Read the model definition and answer for the solid it produces. Units are mm, in the model's axes. A direction names the side the tool comes from. Give positions to 0.01 mm unless a question says otherwise; leave off trailing zeros. Order: outer loops, then holes, each group sorted by start corner. A loop starts at its lowest first (then second) coordinate and runs counter-clockwise, first axis right, second up. Notation, with made-up numbers: M -38.75,-3.5 L -29.75,-3.5 A15 ccw -29.75,17.5 Z; hole C -29.75,87 d1. An arc over 180 degrees is marked long. Write item = value, one per line. Start each with the question number.
from build123d import *

# Parameters (mm, degrees)
BOSS_EXTRUDE1_DEPTH     = 18
CUT_EXTRUDE1_DEPTH      = 18
EXTRUDE_THIN1_DEPTH     = 25
CUT_EXTRUDE2_DEPTH      = 78.777509214
CUT_EXTRUDE2_DEPTH_BACK = 78.777509214
SKETCH3_R               = 2.5
CHAMFER1_SIZE           = 1
CUT_EXTRUDE3_DEPTH      = 67.100990458
CUT_EXTRUDE3_DEPTH_BACK = 67.100990458
SKETCH6_R               = 2.5
CHAMFER3_SIZE           = 1


with BuildPart() as part:
    # Sketch1 → Boss-Extrude1 (new body)
    with BuildSketch(Plane(origin=(0, 0, 0), x_dir=(1, 0, 0), z_dir=(0, 1, 0))):
        with BuildLine():
            Line((40.156887748, -10), (40.156887748, 10))
            Line((40.156887748, 10), (30.5, 20))
            Line((30.5, 20), (-17.5, 20))
            ThreePointArc((-17.5, 20), (-31.64213568, 14.142135567), (-37.5, -1.6e-07))
            ThreePointArc((-37.5, -1.6e-07), (-31.642135567, -14.14213568), (-17.5, -20))
            Line((-17.5, -20), (30.5, -20))
            Line((30.5, -20), (40.156887748, -10))
        make_face()
    extrude(amount=BOSS_EXTRUDE1_DEPTH)

    # Sketch2 → Cut-Extrude1 (cut)
    with BuildSketch(Plane.XZ):
        Polygon((27.5, 5.5), (27.5, -5.5), (23.964466094, -9.035533906), (12.964466094, -9.035533906), (9.428932188, -5.5), (9.428932188, 5.5), (12.964466094, 9.035533906), (23.964466094, 9.035533906), align=None)
    extrude(amount=-CUT_EXTRUDE1_DEPTH, mode=Mode.SUBTRACT)

    # Sketch4 → Extrude-Thin1 (add)
    with BuildSketch(Plane.XZ):
        with BuildLine():
            Line((-17.5, -32), (35.593697795, -32))
            Line((35.593697795, -32), (52.156887748, -14.84831471))
            Line((52.156887748, -14.84831471), (52.156887748, 14.84831471))
            Line((52.156887748, 14.84831471), (35.593697795, 32))
            Line((35.593697795, 32), (-17.5, 32))
            ThreePointArc((-17.5, 32), (-49.5, 0), (-17.5, -32))
        make_face()
        with BuildLine():
            Line((-17.5, -20), (30.5, -20))
            Line((30.5, -20), (40.156887748, -10))
            Line((40.156887748, -10), (40.156887748, 10))
            Line((40.156887748, 10), (30.5, 20))
            Line((30.5, 20), (-17.5, 20))
            ThreePointArc((-17.5, 20), (-37.5, 0), (-17.5, -20))
        make_face(mode=Mode.SUBTRACT)
    extrude(amount=-EXTRUDE_THIN1_DEPTH)

    # Sketch3 → Cut-Extrude2 (cut, two sides: drawn at the far end of the back side and taken through both)
    with BuildSketch(Plane.XY.offset(20).offset(-CUT_EXTRUDE2_DEPTH_BACK)):
        with Locations((18.464466094, 5.5)):
            Circle(SKETCH3_R)
    extrude(amount=CUT_EXTRUDE2_DEPTH + CUT_EXTRUDE2_DEPTH_BACK, mode=Mode.SUBTRACT)

    # Chamfer1
    chamfer1_edges = [part.edges().sort_by_distance(p)[0] for p in [
        (-49.5, 25, 0),
        (9.046848897, 25, 32),
        (43.875292771, 25, 23.424157355),
        (52.156887748, 25, 0),
        (43.875292771, 25, -23.424157355),
        (9.046848897, 25, -32),
        (15.964466094, 5.5, -32),
        (15.964466094, 5.5, 32),
    ]]
    chamfer(chamfer1_edges, length=CHAMFER1_SIZE)

    # Sketch6 → Cut-Extrude3 (cut, two sides: drawn at the far end of the back side and taken through both)
    with BuildSketch(Plane(origin=(0, 25, 0), x_dir=(1, 0, 0), z_dir=(0, 1, 0)).offset(-CUT_EXTRUDE3_DEPTH_BACK)):
        with Locations(Location((0, 25.5, 0), (0, 0, 270))):
            Circle(SKETCH6_R)
        with Locations(Location((0, -25.5, 0), (0, 0, 270))):
            Circle(SKETCH6_R)
        with Locations(Location((45.656887748, 0, 0), (0, 0, 270))):
            Circle(SKETCH6_R)
        with Locations(Location((-43, 0, 0), (0, 0, 270))):
            Circle(SKETCH6_R)
    extrude(amount=CUT_EXTRUDE3_DEPTH + CUT_EXTRUDE3_DEPTH_BACK, mode=Mode.SUBTRACT)

    # Chamfer3
    chamfer3_edges = [part.edges().sort_by_distance(p)[0] for p in [
        (0, 25, -28),
        (0, 25, 23),
        (45.656887748, 25, -2.5),
        (-43, 25, -2.5),
    ]]
    chamfer(chamfer3_edges, length=CHAMFER3_SIZE)


solid = part.part
1) Each of these flat-tipped pins is pushed along its axis until it touches: P1, Ø1, axis at y = 17.5, z = 22, coming from the -X side; P2, Ø6.5, axis at x = 18.46, y = 5.5, coming from the -Z side; P3, Ø3.5, axis at y = 21, z = -1.5, coming from the -X side; P4, Ø4.5, axis at x = 18.46, y = 5.5, coming from the +Z side. Where does it stop, or does it pass through?
2) Find the intervals of material crossed by probe 1 along Z at (x, y) = (0, 9.25); probe 2 along X at (y, z) = (7, 0); probe 3 along X at (y, z) = (18.25, 0), in increasing order. Write a range as [from, to].
3) Find section A-A on z = 0. Determine the outline of the cut face in (x, y).
4) Find section D-D on y = 10.5. Determine the outline of the cut face in (x, z), plus the area to 3 significant figures.
5) Find section B-B on x = 0. Determine the outline of the cut face in (y, z).
6) For a pull along Z with two mould halves and no side action, classify faces 1 (the face through (-49.492, 11.832, 0.704)), 2 (the face through (9, 12, 32)), 3 (the face through (19, 9, -9.036)), 4 (the face through (11.17, 8.87, 7.24)) as pulls with the +Z half, pulls with the -Z half, needs draft (parallel to the pull), parting line crosses it, or undercut.
7) Find section C-C on y = 5.5. Count the separate pieces of the cut face and the enclosed holes in it, plus the area to 3 significant figures.
8) For faces 5 (the face through (-48.65, 24.84, 0.69)), 6 (the face through (6, 21, -20)), 7 (the face through (27.5, 9, 0)), determine the directions among +Z, -Z, +X, -X, +Y, -Y from which every point of the face is accessible in a straight line to the end or side of a thin tool.
Numbers:
q1.P1 = -41.2
q1.P2 = -31.75
q1.P3 = -49.5
q1.P4 = through
q2.probe_1 = [-32, -28], [-23, 23], [28, 32]
q2.probe_2 = [-49.5, -45.5], [-40.5, 9.43], [27.5, 43.16], [48.16, 52.16]
q2.probe_3 = [-49.5, -45.5], [-40.5, -37.5], [40.16, 43.16], [48.16, 52.16]
q3.outline = M -49.5,0 L -45.5,0 L -45.5,24 L -46.5,25 L -48.5,25 L -49.5,24 Z; M -40.5,0 L 9.43,0 L 9.43,18 L -37.5,18 L -37.5,25 L -39.5,25 L -40.5,24 Z; M 27.5,0 L 43.16,0 L 43.16,24 L 42.16,25 L 40.16,25 L 40.16,18 L 27.5,18 Z; M 48.16,0 L 52.16,0 L 52.16,24 L 51.16,25 L 49.16,25 L 48.16,24 Z
q4.outline = M -17.5,-32 L 35.59,-32 L 52.16,-14.85 L 52.16,14.85 L 35.59,32 L -17.5,32 A32 ccw Z; hole C -43,0 d5; hole C 0,-25.5 d5; hole C 0,25.5 d5; hole M 9.43,-5.5 L 12.96,-9.04 L 23.96,-9.04 L 27.5,-5.5 L 27.5,5.5 L 23.96,9.04 L 12.96,9.04 L 9.43,5.5 Z; hole C 45.66,0 d5
q4.area = 5,400 mm2
q5.outline = M 0,-32 L 24,-32 L 25,-31 L 25,-29 L 24,-28 L 0,-28 Z; M 0,-23 L 24,-23 L 25,-22 L 25,-20 L 18,-20 L 18,20 L 25,20 L 25,22 L 24,23 L 0,23 Z; M 0,28 L 24,28 L 25,29 L 25,31 L 24,32 L 0,32 Z
q6.face_1 = parting line crosses it
q6.face_2 = pulls with the +Z half
q6.face_3 = undercut
q6.face_4 = undercut
q7.separate_pieces = 2
q7.enclosed_holes = 4
q7.area = 5,170 mm2
q8.face_5 = -X, +Y
q8.face_6 = +Y
q8.face_7 = +Y, -Y
